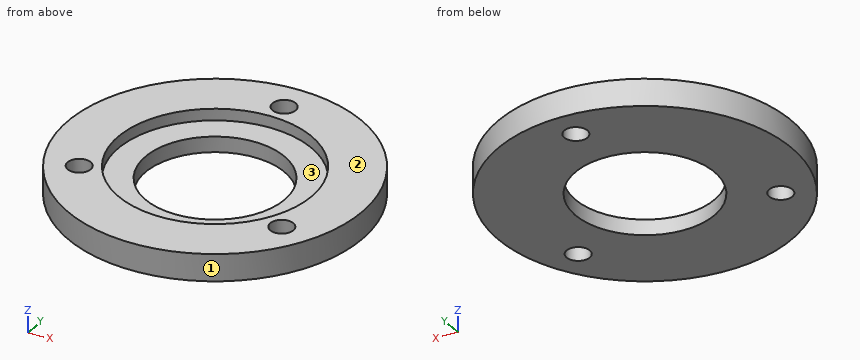
from build123d import *

# Parameters (mm, degrees)
SKETCH1_R               = 19
BOSS_EXTRUDE1_DEPTH     = 2
SKETCH2_R               = 19
SKETCH2_R_2             = 12.5
BOSS_EXTRUDE2_DEPTH     = 1.5
CUT_EXTRUDE1_DEPTH      = 27.944387171
CUT_EXTRUDE1_DEPTH_BACK = 27.944387171
SKETCH3_R               = 9
SKETCH4_R               = 1.5
CUT_EXTRUDE2_DEPTH      = 28.09704781
CIRPATTERN1_COUNT       = 3


with BuildPart() as part:
    # Sketch1 → Boss-Extrude1 (new body)
    with BuildSketch(Plane.XY):
        Circle(SKETCH1_R)
    extrude(amount=BOSS_EXTRUDE1_DEPTH)

    # Sketch2 → Boss-Extrude2 (add)
    with BuildSketch(Plane.XY.offset(2)):
        Circle(SKETCH2_R)
        Circle(SKETCH2_R_2, mode=Mode.SUBTRACT)
    extrude(amount=BOSS_EXTRUDE2_DEPTH)

    # Sketch3 → Cut-Extrude1 (cut, two sides: drawn at the far end of the back side and taken through both)
    with BuildSketch(Plane.XY.offset(2).offset(-CUT_EXTRUDE1_DEPTH_BACK)):
        Circle(SKETCH3_R)
    extrude(amount=CUT_EXTRUDE1_DEPTH + CUT_EXTRUDE1_DEPTH_BACK, mode=Mode.SUBTRACT)

    # Sketch4 → Cut-Extrude2 (cut, symmetric)
    with BuildSketch(Plane.XY):
        with Locations((0, 15)):
            Circle(SKETCH4_R)
    cut_extrude2 = extrude(amount=CUT_EXTRUDE2_DEPTH, both=True, mode=Mode.SUBTRACT)

    # CirPattern1: Cut-Extrude2 ×3 about axis
    cirpattern1_axis = Axis((0, 0, 0), (0, 0, 1))
    for i in range(1, CIRPATTERN1_COUNT):
        add(cut_extrude2.rotate(cirpattern1_axis, i * 360 / CIRPATTERN1_COUNT), mode=Mode.SUBTRACT)


solid = part.part
Verification items for the finished model (mm, model axes). Face numbers are marked on the shaded views. Round coordinates to 2 decimals unless told otherwise and drop trailing zeros. Order: outer loops, then holes, each group sorted by start corner. A loop starts at its lowest first (then second) coordinate and runs counter-clockwise, first axis right, second up. Notation, with made-up numbers: (45, 43) -> (73, 43) arc R5 ccw to (73, 52) -> close; hole circle Ø4 at (23.5, 27). An arc over 180 degrees is marked (long way). Put each result on its own line as item: value.
1) Section check D-D (z = 2.6). Record the cut outline in (x, y), then the cut area to 3 significant figures.
Final values:
outline: circle Ø38 at (0, 0); hole circle Ø3 at (-12.99, -7.5); hole circle Ø25 at (0, 0); hole circle Ø3 at (0, 15); hole circle Ø3 at (12.99, -7.5)
area: 622 mm^2
2) Depth check by flat-ended pin: pin 1 (20.5 mm diameter, centred on x = 0, y = 0, fed in from +Z); pin 2 (1.8 mm diameter, centred on x = 12.99, y = -7.5, fed in from -Z); pin 3 (1 mm diameter, centred on x = -15, z = 1, fed in from -Y); pin 4 (1.5 mm diameter, centred on x = -6, z = 1.5, fed in from +Y). Enter the tip coordinate at first touch or a pass-through.
Final values:
pin 1: stops at z = 2
pin 2: passes through
pin 3: stops at y = -12.28
pin 4: stops at y = 18.26
3) Mould release check, pull along Y, two halves, no side actions. Record for the marked faces 1, 2 and 3: +Y half, -Y half, draft (parallel to the pull), parting line (faces both ways), or undercut.
Final values:
face 1: parting line
face 2: draft
face 3: undercut
4) Material ranges on line 1 (Y direction, x = 0, z = 1.1); line 2 (Y direction, x = 0, z = 2.05); line 3 (Y direction, x = -5.5, z = 2.1), recorded low to high.
Final values:
line 1: y = -19 to -9, 9 to 13.5, 16.5 to 19
line 2: y = -19 to -12.5, 12.5 to 13.5, 16.5 to 19
line 3: y = -18.19 to -11.22, 11.22 to 18.19
5) Section check C-C (x = 4). Record the cut outline in (y, z).
Final values:
outline: (-18.57, 0) -> (-8.06, 0) -> (-8.06, 2) -> (-11.84, 2) -> (-11.84, 3.5) -> (-18.57, 3.5) -> close; (8.06, 0) -> (18.57, 0) -> (18.57, 3.5) -> (11.84, 3.5) -> (11.84, 2) -> (8.06, 2) -> close
6) Section check B-B (y = 0). Record the cut outline in (x, z).
Final values:
outline: (-19, 0) -> (-9, 0) -> (-9, 2) -> (-12.5, 2) -> (-12.5, 3.5) -> (-19, 3.5) -> close; (9, 0) -> (19, 0) -> (19, 3.5) -> (12.5, 3.5) -> (12.5, 2) -> (9, 2) -> close
7) Section check A-A (x = 0). Record the cut outline in (y, z).
Final values:
outline: (-19, 0) -> (-9, 0) -> (-9, 2) -> (-12.5, 2) -> (-12.5, 3.5) -> (-19, 3.5) -> close; (9, 0) -> (13.5, 0) -> (13.5, 3.5) -> (12.5, 3.5) -> (12.5, 2) -> (9, 2) -> close; (16.5, 0) -> (19, 0) -> (19, 3.5) -> (16.5, 3.5) -> close
